Autodesk Inventor part; units mm, degrees
ref_plane "YZ Plane" through (0, 0, 0) normal (1, 0, 0) x (0, 1, 0)
ref_plane "XZ Plane" through (0, 0, 0) normal (0, 1, 0) x (-1, 0, 0)
ref_plane "XY Plane" through (0, 0, 0) normal (0, 0, 1) x (1, 0, 0)
sketch "Sketch1" plane through (0, 0, 0) normal (0, 0, 1) x (1, 0, 0)
  circle A0 centre (0, 0) radius 38
  line L0 (0, -38) -> (1000, -38)
  line L1 (1000, -38) -> (1000, -18)
  line L2 (1000, -18) -> (0, -18)
  line L3 (0, -18) -> (0, -38)
  line L4 (0, 38) -> (68, 38)
  line L5 (68, 38) -> (68, 18)
  line L6 (68, 18) -> (0, 18)
  line L7 (0, 18) -> (0, 38)
  circle A1 centre (0, 0) radius 18
  dimension "d0" = 76
  dimension "d1" = 20
  dimension "d2" = 20
  dimension "d4" = 1000
  dimension "d7" = 68
extrude "Extrusion1" add sketch "Sketch1" along normal blind 39 contours L7 A1 L3 A0 | L4 L5 L6 A0 | A0 L6 L7 | L3 L2 A0 | A0 L2 L1 L0
properties part number "J15BF.1.30"
Can you work these out from the model? Positions are in its coordinate system, mm. A direction names the side the tool comes from. Coordinates: 2 decimals unless noted, no trailing zeros. Loops run counter-clockwise (first coordinate to the right, second up) from the corner with the lowest first, then second, coordinate; pieces in that order, holes last.
1) I need wall thicknesses on probe 1 along Y at (x, z) = (668, 14.5); probe 2 along Y at (x, z) = (66, 6.5); probe 3 along X at (y, z) = (1, 29). Which ranges of each line are inside material? Lowest first, please.
2) Which directions (+Z, -Z, +X, -X, +Y, -Y) give clear straight access to the entire face, cutting with the end or side of a thin tool? Please do faces 1 (the flat face through (34, 18, 19)), 2 (the flat face through (68, 28, 19)), 3 (the flat face through (402, -22, 39)).
3) Imagine slicing it at B-B on x = 437.5. List the corners of the cut face in (y, z) for me.
4) Imagine slicing it at A-A on z = 10. List the corners of the cut face in (x, y) for me.
5) For pin 1 (1 mm diameter, centred on y = -7.5, z = 4, fed in from -X); pin 2 (3 mm diameter, centred on x = 173, z = 29, fed in from +Y); pin 3 (3 mm diameter, centred on y = 21, z = 25, fed in from -X); pin 4 (12 mm diameter, centred on x = 613.5, y = -7, fed in from -Z) (3 decimals), each with a flat end and sliding along its axis, tell me the tip position at first contact or that it passes through.
Completed:
1. probe 1: y = -38 to -18
1. probe 2: y = -38 to -18, 18 to 38
1. probe 3: x = -37.99 to -17.97
2. face 1: +Z, -Z, +X
2. face 2: +Z, -Z, +X, +Y
2. face 3: +Z, +X, -X, +Y, -Y
3. outline: (-38, 0) - (-18, 0) - (-18, 39) - (-38, 39) - close
4. outline: (0, -38) - (1000, -38) - (1000, -18) - (0, -18) arc R18 cw to (0, 18) - (68, 18) - (68, 38) - (0, 38) arc R38 ccw to start
5. pin 1: stops at x = -37.35
5. pin 2: stops at y = -18
5. pin 3: stops at x = -32.62
5. pin 4: passes through
